The figure shows three views and two pictorial views of one solid part (mm, origin at its lowest corner). Answer the questions. Coordinates: 2 decimals unless noted, no trailing zeros. Write each loop counter-clockwise with the first axis right and the second up, starting at its lowest first coordinate (ties: lowest second). Pieces come first, ordered by that corner, then holes.
Item 1: Section B-B (x = 22.5) is taken. Give the vertices of the cut face in (y, z) (3 decimals), then the cut area to 3 significant figures.
Item 2: Each of these flat-tipped pins is pushed along its axis until it touches: P1, Ø5, axis at y = 6, z = 46.5, coming from the +X side (3 decimals); P2, Ø1, axis at x = 46, y = 2.5, coming from the -Z side (3 decimals). Where does it stop, or does it pass through?
Item 3: Section A-A (y = 4.5) is taken. Give the vertices of the cut face in (x, z) (3 decimals).
Item 4: Straight lines are drawn through the part: probe 1 along X at (y, z) = (6.25, 64) (3 decimals); probe 2 along X at (y, z) = (1.25, 42) (3 decimals); probe 3 along Z at (x, y) = (65.5, 7.25) (3 decimals). For each, find the intervals that lie inside material, in ascending order.
Item 5: Section C-C (z = 14.5) is taken. Give the vertices of the cut face in (x, y) (3 decimals).
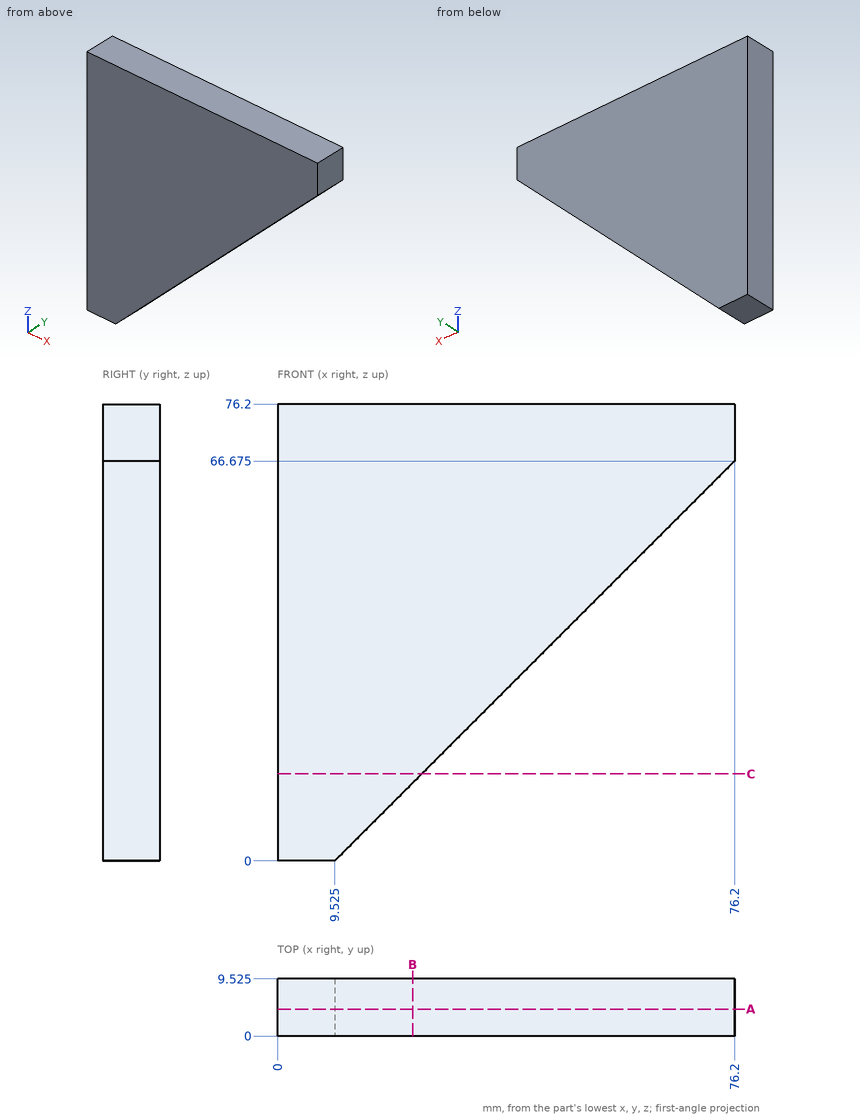
Established:
1. outline: (0, 12.975) - (9.525, 12.975) - (9.525, 76.2) - (0, 76.2) - close
1. area: 602 mm2
2. P1: stops at x = 58.525
2. P2: stops at z = 35.975
3. outline: (0, 0) - (9.525, 0) - (76.2, 66.675) - (76.2, 76.2) - (0, 76.2) - close
4. probe 1: x = 0 to 73.525
4. probe 2: x = 0 to 51.525
4. probe 3: z = 55.975 to 76.2
5. outline: (0, 0) - (24.025, 0) - (24.025, 9.525) - (0, 9.525) - close
